Source: CAD feature listing. Evaluate the final solid. Frame: model axes, mm. Give positions to 0.01 mm unless a question says otherwise; leave off trailing zeros. Loops run counter-clockwise (first coordinate to the right, second up) from the corner with the lowest first, then second, coordinate; pieces in that order, holes last.
```python
from build123d import *

# Parameters (mm, degrees)
EXTRUDE_1_DEPTH     = 4
FILLET_1_R          = 2
CUT_EXTRUDE_2_DEPTH = 64.492631813


with BuildPart() as part:
    # 草图2 → 凸台-拉伸1 (new body)
    with BuildSketch(Plane(origin=(0, 0, 0), x_dir=(1, 0, 0), z_dir=(0, 1, 0))):
        with BuildLine():
            Line((-24.75, -4), (-36, -4))
            ThreePointArc((-36, -4), (-38.516568808, -3.109160889), (-39.912208656, -0.833440718))
            ThreePointArc((-39.912208656, -0.833440718), (0, 48.477143514), (39.912208656, -0.833440718))
            ThreePointArc((39.912208656, -0.833440718), (38.516568808, -3.109160889), (36, -4))
            Line((36, -4), (24.75, -4))
            ThreePointArc((24.75, -4), (21.21885665, -1.879102616), (21.432309646, 2.234486679))
            ThreePointArc((21.432309646, 2.234486679), (0, 42.509326923), (-21.432309646, 2.234486679))
            ThreePointArc((-21.432309646, 2.234486679), (-21.21885665, -1.879102616), (-24.75, -4))
        make_face()
        with BuildLine():
            Line((-36, 1.65), (-24.75, 1.65))
            ThreePointArc((-24.75, 1.65), (-23.1, 0), (-24.75, -1.65))
            Line((-24.75, -1.65), (-36, -1.65))
            ThreePointArc((-36, -1.65), (-37.65, 0), (-36, 1.65))
        make_face(mode=Mode.SUBTRACT)
        with BuildLine():
            Line((36, 1.65), (24.75, 1.65))
            ThreePointArc((24.75, 1.65), (23.1, 0), (24.75, -1.65))
            Line((24.75, -1.65), (36, -1.65))
            ThreePointArc((36, -1.65), (37.65, 0), (36, 1.65))
        make_face(mode=Mode.SUBTRACT)
    extrude(amount=EXTRUDE_1_DEPTH)

    # 圆角1
    fillet_1_edges = [part.edges().sort_by_distance(p)[0] for p in [
        (-38.516568808, 0, 3.109160889),
        (0, 0, -48.477143514),
        (38.516568808, 0, 3.109160889),
        (30.375, 0, 4),
        (21.21885665, 0, 1.879102616),
        (0, 0, -42.509326923),
        (-21.21885665, 0, 1.879102616),
        (-21.21885665, 4, 1.879102616),
        (-30.375, 4, 4),
        (-38.516568808, 4, 3.109160889),
        (0, 4, -48.477143514),
        (38.516568808, 4, 3.109160889),
        (30.375, 4, 4),
        (21.21885665, 4, 1.879102616),
        (-30.375, 0, 4),
        (0, 4, -42.509326923),
    ]]
    fillet(fillet_1_edges, radius=FILLET_1_R - 0.0001)  # a hair under: the kernel refuses the full size

    # 草图4 → 切除-拉伸2 (cut, through all)
    with BuildSketch(Plane(origin=(0, 4, 0), x_dir=(1, 0, 0), z_dir=(0, 1, 0))):
        with BuildLine():
            Line((-34.872154706, 3.65), (-29.437290433, 3.65))
            ThreePointArc((-29.437290433, 3.65), (-28.334992254, 4.233967388), (-28.198977603, 5.473959002))
            ThreePointArc((-28.198977603, 5.473959002), (-30.310084994, 18.017081432), (-27.0940075, 30.323321324))
            ThreePointArc((-27.0940075, 30.323321324), (-27.266499401, 30.966568064), (-27.925113784, 30.867841575))
            ThreePointArc((-27.925113784, 30.867841575), (-34.578408784, 18.729054984), (-36.204488684, 4.982333979))
            ThreePointArc((-36.204488684, 4.982333979), (-35.814257097, 4.040231588), (-34.872154706, 3.65))
        make_face()
    cut_extrude_2 = extrude(amount=-CUT_EXTRUDE_2_DEPTH, mode=Mode.SUBTRACT)

    # 镜向1: 切除-拉伸2 across plane
    add(cut_extrude_2.mirror(Plane(origin=(0, 0, 0), x_dir=(0, 0, 1), z_dir=(1, 0, 0))), mode=Mode.SUBTRACT)


solid = part.part
```
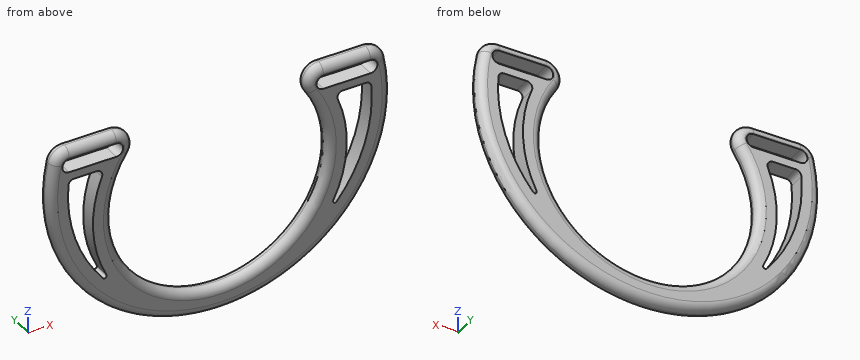
(1) First-contact query: pin 1 (12 mm diameter, centred on x = -30.5, z = -3, fed in from -Y); pin 2 (1.2 mm diameter, centred on x = 31, y = 3, fed in from -Z). Flat tips, straight axial feed; report the tip coordinate or a pass-through.
A:
pin 1: stops at y = 0
pin 2: stops at z = -34.61
(2) Section C-C, the plane z = -22.5. Count the separate pieces of the cut face and the enclosed holes in it, then the cut area to 3 significant figures.
A:
separate pieces: 4
enclosed holes: 0
area: 68.6 mm2
(3) Section B-B, the plane y = 1.2. Return the cut outline in (x, z).
A:
outline: (-39.75, 0.8) arc R40.64 ccw (long way) to (39.75, 0.8) arc R3.83 ccw to (36, 3.83) - (24.75, 3.83) arc R3.83 ccw to (21.57, -2.14) arc R26.01 cw (long way) to (-21.57, -2.14) arc R3.83 ccw to (-24.75, 3.83) - (-36, 3.83) arc R3.83 ccw to start; hole (-36.2, -4.98) arc R36.3 ccw to (-27.93, -30.87) arc R0.5 ccw to (-27.09, -30.32) arc R30.34 cw to (-28.2, -5.47) arc R1.33 ccw to (-29.44, -3.65) - (-34.87, -3.65) arc R1.33 ccw to start; hole (-36, -1.65) - (-24.75, -1.65) arc R1.65 ccw to (-24.75, 1.65) - (-36, 1.65) arc R1.65 ccw to start; hole (24.75, -1.65) - (36, -1.65) arc R1.65 ccw to (36, 1.65) - (24.75, 1.65) arc R1.65 ccw to start; hole (27.09, -30.32) arc R0.5 ccw to (27.93, -30.87) arc R36.3 ccw to (36.2, -4.98) arc R1.33 ccw to (34.87, -3.65) - (29.44, -3.65) arc R1.33 ccw to (28.2, -5.47) arc R30.34 cw to start
(4) Ray query, line 1 along X through (y, z) = (1.8, -18.5); line 2 along X through (y, z) = (2.2, -5); line 3 along Z through (x, y) = (0, 2.05). Return the intervals inside material, ascending.
A:
line 1: x = -39.33 to -34.65, -30.28 to -25.79, 25.79 to 30.28, 34.65 to 39.33
line 2: x = -40.71 to -36.21, -28.11 to -23.07, 23.07 to 28.11, 36.21 to 40.71
line 3: z = -48.48 to -42.51
